Could you check a few things on this drawing? It's one solid part, dimensions in mm from its lowest x, y, z. A direction names the side the tool comes from. Give positions to 0.01 mm unless a question says otherwise; leave off trailing zeros. Order: outer loops, then holes, each group sorted by start corner. A loop starts at its lowest first (then second) coordinate and runs counter-clockwise, first axis right, second up. Notation, with made-up numbers: (12, 37.5) -> (37, 37.5) arc R5 cw to (37, 46.5) -> close; hole circle Ø10 at (-26.5, 52). An arc over 180 degrees is marked (long way). Answer as CSV lines item,"result".
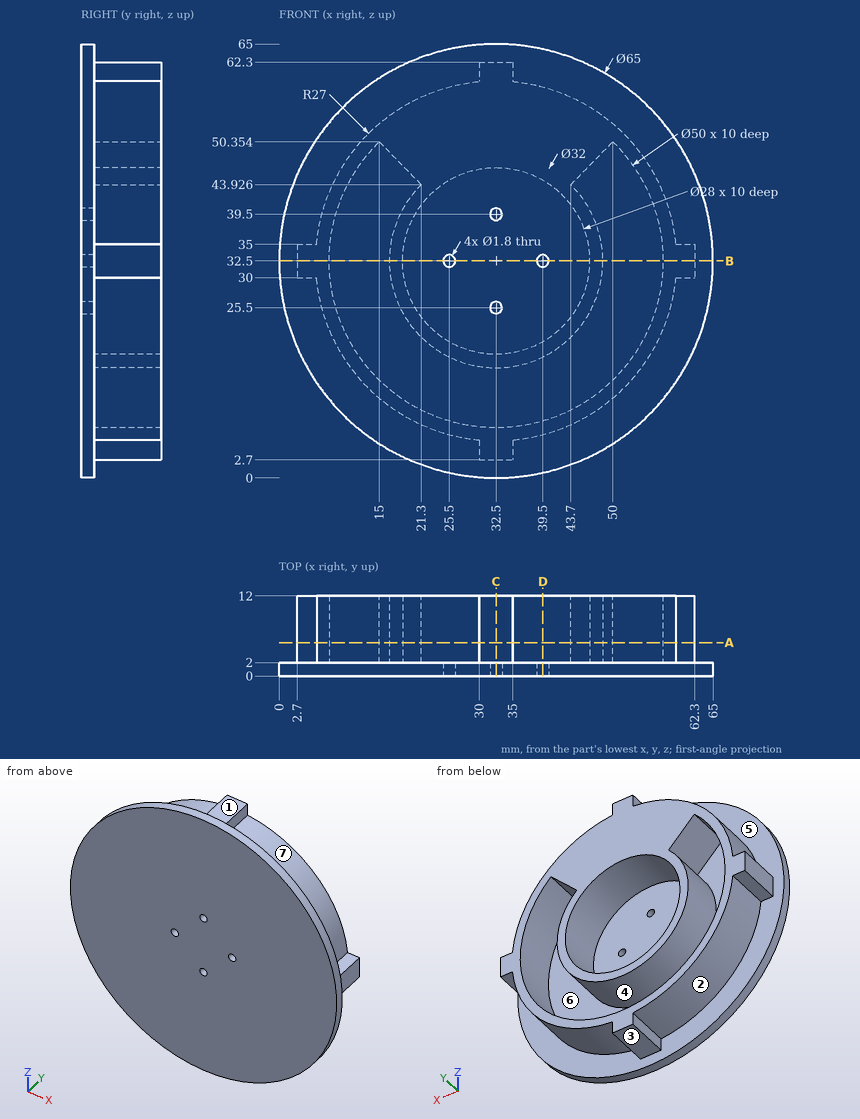
Item 1: Imagine slicing it at D-D, the plane x = 39.5. Please give me the cut outline in (y, z) (1 decimal).
Numbers:
outline,"(0, 0.8) -> (2, 0.8) -> (2, 6.4) -> (12, 6.4) -> (12, 8.5) -> (2, 8.5) -> (2, 18.1) -> (12, 18.1) -> (12, 20.4) -> (2, 20.4) -> (2, 31.6) -> (0, 31.6) -> close; (0, 33.4) -> (2, 33.4) -> (2, 44.6) -> (12, 44.6) -> (12, 58.6) -> (2, 58.6) -> (2, 64.2) -> (0, 64.2) -> close"
Item 2: Imagine slicing it at B-B, the plane z = 32.5. Please give me the cut outline in (x, y).
Numbers:
outline,"(0, 0) -> (24.6, 0) -> (24.6, 2) -> (18.5, 2) -> (18.5, 12) -> (16.5, 12) -> (16.5, 2) -> (7.5, 2) -> (7.5, 12) -> (2.7, 12) -> (2.7, 2) -> (0, 2) -> close; (26.4, 0) -> (38.6, 0) -> (38.6, 2) -> (26.4, 2) -> close; (40.4, 0) -> (65, 0) -> (65, 2) -> (62.3, 2) -> (62.3, 12) -> (57.5, 12) -> (57.5, 2) -> (48.5, 2) -> (48.5, 12) -> (46.5, 12) -> (46.5, 2) -> (40.4, 2) -> close"
Item 3: Imagine slicing it at A-A, the plane y = 5. Please give me the cut outline in (x, z).
Numbers:
outline,"(2.7, 30) -> (5.62, 30) arc R27 ccw to (30, 5.62) -> (30, 2.7) -> (35, 2.7) -> (35, 5.62) arc R27 ccw to (59.38, 30) -> (62.3, 30) -> (62.3, 35) -> (59.38, 35) arc R27 ccw to (35, 59.38) -> (35, 62.3) -> (30, 62.3) -> (30, 59.38) arc R27 ccw to (5.62, 35) -> (2.7, 35) -> close; hole (15, 50.35) arc R25 ccw (long way) to (50, 50.35) -> (43.7, 43.93) arc R16 cw (long way) to (21.3, 43.93) -> close; hole circle Ø28 at (32.5, 32.5)"
Item 4: For the marked faces 1, 2, 3 and 4, which set-ups out of +Z, -Z, +X, -X, +Y, -Y let a thin tool reach every point of the face, with its end or its side?
Numbers:
face 1,"+Z, +X, -X, +Y"
face 2,"-Z, -X, +Y"
face 3,"-Z, +X, -X, +Y"
face 4,"+Y"
Item 5: For pin 1 (1.5 mm diameter, centred on y = 6, z = 61.5, fed in from +X); pin 2 (1 mm diameter, centred on x = 9, y = 3, fed in from -Z); pin 3 (1 mm diameter, centred on x = 30.5, z = 10.5, fed in from +Y); pin 4 (1.1 mm diameter, centred on x = 32.5, z = 39.5, fed in from -Y), each with a flat end and sliding along its axis, tell me the tip position at first contact or that it passes through.
Numbers:
pin 1,"stops at x = 35"
pin 2,"stops at z = 18.36"
pin 3,"stops at y = 2"
pin 4,"passes through"
Item 6: We'd pull the mould along X, two halves only. Please class the marked faces 5, 6 and 7: released by +X, released by -X, zero draft, split by the parting line, or undercut.
Numbers:
face 5,"zero draft"
face 6,"undercut"
face 7,"released by +X"
Item 7: Imagine slicing it at C-C, the plane x = 32.5. Please give me the cut outline in (y, z), then the cut area to 3 significant figures.
Numbers:
outline,"(0, 0) -> (2, 0) -> (2, 2.7) -> (12, 2.7) -> (12, 7.5) -> (2, 7.5) -> (2, 16.5) -> (12, 16.5) -> (12, 18.5) -> (2, 18.5) -> (2, 24.6) -> (0, 24.6) -> close; (0, 26.4) -> (2, 26.4) -> (2, 38.6) -> (0, 38.6) -> close; (0, 40.4) -> (2, 40.4) -> (2, 46.5) -> (12, 46.5) -> (12, 62.3) -> (2, 62.3) -> (2, 65) -> (0, 65) -> close"
area,"349 mm²"
Item 8: Please list where these lines run through material, in increasing order: line 1 along X through (y, z) = (6.25, 32.5); line 2 along X through (y, z) = (0.4, 32.5); line 3 along Z through (x, y) = (36.5, 8.25).
Numbers:
line 1,"x = 2.7 to 7.5, 16.5 to 18.5, 46.5 to 48.5, 57.5 to 62.3"
line 2,"x = 0 to 24.6, 26.4 to 38.6, 40.4 to 65"
line 3,"z = 5.8 to 7.82, 17.01 to 19.08, 45.92 to 59.2"
